Here's how the part is built. I have some questions about the finished solid (model axes, mm). Round coordinates to 2 decimals unless told otherwise and drop trailing zeros. Write each loop counter-clockwise with the first axis right and the second up, starting at its lowest first coordinate (ties: lowest second). Pieces come first, ordered by that corner, then holes. Notation, with made-up numbers: (15.25, -37.5) -> (24.25, -37.5) arc R23 cw to (24.25, 0.5) -> close; hole circle Ø3 at (88, 72). An arc over 180 degrees is marked (long way). Put each result on its own line as item: value. Start each with the question number.
1. We'd pull the mould along X, two halves only. Please class faces 1 (the face through (-51, 6.4, 1.1)), 2 (the face through (-52.87, 8, 1)), 3 (the face through (-49, 16.174, 1)): +X half, -X half, draft (parallel to the pull), parting line (faces both ways), or undercut.
2. I need wall thicknesses on probe 1 along Y at (x, z) = (-49, 0.4); probe 2 along Y at (x, z) = (-51, 1.8); probe 3 along X at (y, z) = (9, 1.4). Which ranges of each line are inside material? Lowest first, please. Write a range as from..to.
3. Suppose I cut it at A-A (z = 0.7). Please give me the cut outline in (x, y).
```python
from build123d import *

# Parameters (mm, degrees)
F0_W     = 8
F0_H     = 16.1739148081
F1_DEPTH = 2.5
F2_SIZE  = 2
F3_R     = 5
F4_R     = 0.5
F5_R     = 2.719161288
F6_DEPTH = 25
F7_R     = 0.25


with BuildPart() as f1:
    # F0 (on Top) → F1 (new body)
    with BuildSketch(Plane.XY):
        with Locations((-48.8695710708, 8.0869574041)):
            Rectangle(F0_W, F0_H)
    extrude(amount=F1_DEPTH)

    # F2
    f2_edges = [f1.edges().sort_by_distance(p)[0] for p in [
        (-44.869571, 0, 1.25),
        (-52.869571, 0, 1.25),
        (-44.869571, 16.173915, 1.25),
        (-52.869571, 16.173915, 1.25),
    ]]
    chamfer(f2_edges, length=F2_SIZE)

    # F3
    f3_edges = [f1.edges().sort_by_distance(p)[0] for p in [
        (-52.869571, 14.173915, 1.25),
        (-52.869571, 2, 1.25),
        (-44.869571, 2, 1.25),
        (-44.869571, 14.173915, 1.25),
    ]]
    fillet(f3_edges, radius=F3_R)

    # F4
    f4_edges = [f1.edges().sort_by_distance(p)[0] for p in [
        (-50.869571, 16.173915, 1.25),
        (-46.869571, 16.173915, 1.25),
        (-46.869571, 0, 1.25),
        (-50.869571, 0, 1.25),
    ]]
    fillet(f4_edges, radius=F4_R)

    # F5 (on face) → F6 (cut)
    with BuildSketch(Plane.XY.offset(2.5)):
        with Locations((-48.8695710708, 8.0869574041)):
            Circle(F5_R)
    extrude(amount=-F6_DEPTH, mode=Mode.SUBTRACT)

    # F7
    f7_edges = [f1.edges().sort_by_distance(p)[0] for p in [
        (-51.588732, 8.086957, 2.5),
        (-52.869571, 8.086957, 2.5),
    ]]
    fillet(f7_edges, radius=F7_R)


solid = f1.part
```
Verdict:
1. face 1: undercut
1. face 2: -X half
1. face 3: draft
2. probe 1: y = 0..5.37, 10.8..16.17
2. probe 2: y = 0.13..6.4, 9.78..16.04
2. probe 3: x = -52.87..-51.43, -46.31..-44.87
3. outline: (-52.87, 4.07) arc R5 ccw to (-51.41, 0.54) -> (-51.02, 0.15) arc R0.5 ccw to (-50.66, 0) -> (-47.08, 0) arc R0.5 ccw to (-46.72, 0.15) -> (-46.33, 0.54) arc R5 ccw to (-44.87, 4.07) -> (-44.87, 12.1) arc R5 ccw to (-46.33, 15.64) -> (-46.72, 16.03) arc R0.5 ccw to (-47.08, 16.17) -> (-50.66, 16.17) arc R0.5 ccw to (-51.02, 16.03) -> (-51.41, 15.64) arc R5 ccw to (-52.87, 12.1) -> close; hole circle Ø5.44 at (-48.87, 8.09)
